from build123d import *

# Parameters (mm, degrees)
EXTRUDE_1_DEPTH     = 26
EXTRUDE_2_DEPTH     = 19
FILLET_1_R          = 10
EXTRUDE_3_DEPTH     = 2
SKETCH_5_W          = 161
SKETCH_5_H          = 6
CUT_EXTRUDE_1_DEPTH = 52
SKETCH_7_W          = 20
SKETCH_7_H          = 20
CUT_EXTRUDE_2_DEPTH = 72
SKETCH_8_W          = 20
SKETCH_8_H          = 20
CUT_EXTRUDE_3_DEPTH = 72
CUT_EXTRUDE_4_DEPTH = 362
SKETCH_9_W          = 9
SKETCH_9_H          = 9
EXTRUDE_4_DEPTH     = 15
EXTRUDE_5_DEPTH     = 20


with BuildPart() as part:
    # Sketch 1 → Extrude 1 (new body)
    with BuildSketch(Plane.XY):
        Polygon((-168, 0), (168, 0), (183, 0), (183, -340), (168, -340), (168, -20), (-168, -20), (-168, -340), (-183, -340), (-183, 0), align=None)
    extrude(amount=EXTRUDE_1_DEPTH)

    # Sketch 1_4 → Extrude 2 (add)
    with BuildSketch(Plane.XY):
        Polygon((172, 0), (168, 0), (168, -20), (168, -340), (172, -340), align=None)
        Polygon((-168, -20), (-168, 0), (-172, 0), (-172, -340), (-168, -340), align=None)
    extrude(amount=-EXTRUDE_2_DEPTH)

    # Fillet 1
    fillet_1_edges = [part.edges().sort_by_distance(p)[0] for p in [
        (170, 0, -19),
        (170, -340, -19),
        (-170, -340, -19),
        (-170, 0, -19),
    ]]
    fillet(fillet_1_edges, radius=FILLET_1_R)

    # Sketch 3 → Extrude 3 (add)
    with BuildSketch(Plane.ZY.offset(-168)):
        with BuildLine():
            Line((-12, -339.539392014), (-12, -0.460607986))
            ThreePointArc((-12, -0.460607986), (-13.02408013, -0.845395743), (-14, -1.339745962))
            Line((-14, -1.339745962), (-14, -338.660254038))
            ThreePointArc((-14, -338.660254038), (-13.02408013, -339.154604257), (-12, -339.539392014))
        make_face()
    extrude_3 = extrude(amount=EXTRUDE_3_DEPTH)

    # Mirror 1: Extrude 3 across plane
    add(extrude_3.mirror(Plane(origin=(0, 0, 0), x_dir=(0, 0, 1), z_dir=(1, 0, 0))))

    # Sketch 5 → Cut-Extrude 1 (cut)
    with BuildSketch(Plane(origin=(0, 0, 0), x_dir=(1, 0, 0), z_dir=(0, 1, 0))):
        with Locations((-87.5, -3)):
            Rectangle(SKETCH_5_W, SKETCH_5_H)
        with Locations((87.5, -3)):
            Rectangle(SKETCH_5_W, SKETCH_5_H)
    extrude(amount=-CUT_EXTRUDE_1_DEPTH, mode=Mode.SUBTRACT)

    # Sketch 7 → Cut-Extrude 2 (cut)
    with BuildSketch(Plane.ZY.offset(-168)):
        with BuildLine():
            Line((26, -340), (26, -20))
            Line((26, -20), (6, -20))
            Line((6, -20), (6, 0))
            Line((6, 0), (-9, 0))
            ThreePointArc((-9, 0), (-10.517576993, -0.115822742), (-12, -0.460607986))
            Line((-12, -0.460607986), (-12, -339.539392014))
            ThreePointArc((-12, -339.539392014), (-10.517576993, -339.884177258), (-9, -340))
            Line((-9, -340), (26, -340))
        make_face()
        with BuildLine():
            Line((-14, -338.660254038), (-14, -1.339745962))
            ThreePointArc((-14, -1.339745962), (-17.660254038, -5), (-19, -10))
            Line((-19, -10), (-19, -330))
            ThreePointArc((-19, -330), (-17.660254038, -335), (-14, -338.660254038))
        make_face()
        with BuildLine():
            ThreePointArc((-12, -0.460607986), (-13.02408013, -0.845395743), (-14, -1.339745962))
            Line((-14, -1.339745962), (-14, -338.660254038))
            ThreePointArc((-14, -338.660254038), (-13.02408013, -339.154604257), (-12, -339.539392014))
            Line((-12, -339.539392014), (-12, -0.460607986))
        make_face()
        with Locations((16, -10)):
            Rectangle(SKETCH_7_W, SKETCH_7_H)
    extrude(amount=-CUT_EXTRUDE_2_DEPTH, mode=Mode.SUBTRACT)


with BuildPart() as cut_extrude_2_piece_1:
    # of the separate pieces the step leaves, piece 1, a body of its own (cut_extrude_2_pieces)
    add(part.part.solids().sort_by_distance((168, 0, 26))[0])

    # Sketch 8 → Cut-Extrude 3 (cut)
    with BuildSketch(Plane(origin=(-168, 0, 0), x_dir=(0, 0, -1), z_dir=(1, 0, 0))):
        with BuildLine():
            Line((9, 0), (-6, 0))
            Line((-6, 0), (-6, -20))
            Line((-6, -20), (-26, -20))
            Line((-26, -20), (-26, -340))
            Line((-26, -340), (9, -340))
            ThreePointArc((9, -340), (10.517576993, -339.884177258), (12, -339.539392014))
            Line((12, -339.539392014), (12, -0.460607986))
            ThreePointArc((12, -0.460607986), (10.517576993, -0.115822742), (9, 0))
        make_face()
        with Locations((-16, -10)):
            Rectangle(SKETCH_8_W, SKETCH_8_H)
    extrude(amount=-CUT_EXTRUDE_3_DEPTH, mode=Mode.SUBTRACT)


with BuildPart() as cut_extrude_2_piece_2:
    # of the separate pieces the step leaves, piece 2, a body of its own (cut_extrude_2_pieces)
    add(part.part.solids().sort_by_distance((168, -339.539392014, -12))[0])


with BuildPart() as cut_extrude_3_piece_1:
    # of the separate pieces the step leaves, piece 1, a body of its own (cut_extrude_3_pieces)
    add(cut_extrude_2_piece_1.part.solids().sort_by_distance((-168, 0, 26))[0])

    # Sketch 9 → Extrude 4 (add)
    with BuildSketch(Plane(origin=(168, 0, 0), x_dir=(0, 0, -1), z_dir=(1, 0, 0))):
        with Locations((-21.5, -15.5)):
            Rectangle(SKETCH_9_W, SKETCH_9_H)
    extrude_4 = extrude(amount=EXTRUDE_4_DEPTH)

    # Mirror 2: Extrude 4 across plane
    add(extrude_4.mirror(Plane(origin=(0, 0, 0), x_dir=(0, 0, 1), z_dir=(1, 0, 0))))

    # Sketch 10 → Extrude 5 (add)
    with BuildSketch(Plane.XY.offset(26)):
        Polygon((168, -20), (162, -20), (168, -26), align=None)
    extrude_5 = extrude(amount=-EXTRUDE_5_DEPTH)

    # Mirror 3: Extrude 5 across plane
    add(extrude_5.mirror(Plane(origin=(0, 0, 0), x_dir=(0, 0, 1), z_dir=(1, 0, 0))))


with BuildPart() as cut_extrude_3_piece_2:
    # of the separate pieces the step leaves, piece 2, a body of its own (cut_extrude_3_pieces)
    add(cut_extrude_2_piece_1.part.solids().sort_by_distance((-172, -0.460607986, -12))[0])


with BuildPart() as cut_extrude_4_tool:
    # Sketch 7_3 → Cut-Extrude 4 (new body)
    with BuildSketch(Plane.ZY.offset(-168)):
        with BuildLine():
            Line((-14, -338.660254038), (-14, -1.339745962))
            ThreePointArc((-14, -1.339745962), (-17.660254038, -5), (-19, -10))
            Line((-19, -10), (-19, -330))
            ThreePointArc((-19, -330), (-17.660254038, -335), (-14, -338.660254038))
        make_face()
        with BuildLine():
            ThreePointArc((-12, -0.460607986), (-13.02408013, -0.845395743), (-14, -1.339745962))
            Line((-14, -1.339745962), (-14, -338.660254038))
            ThreePointArc((-14, -338.660254038), (-13.02408013, -339.154604257), (-12, -339.539392014))
            Line((-12, -339.539392014), (-12, -0.460607986))
        make_face()
    extrude(amount=CUT_EXTRUDE_4_DEPTH)


with BuildPart() as cut_extrude_2_piece_2_1:
    add(cut_extrude_2_piece_2.part)

    # Cut-Extrude 4: cut by cut_extrude_4_tool
    add(cut_extrude_4_tool.part, mode=Mode.SUBTRACT)


with BuildPart() as cut_extrude_3_piece_2_1:
    add(cut_extrude_3_piece_2.part)

    # Cut-Extrude 4: cut by cut_extrude_4_tool
    add(cut_extrude_4_tool.part, mode=Mode.SUBTRACT)


solid = cut_extrude_3_piece_1.part
Verification items for the finished model (mm, model axes). A direction names the side the tool comes from. Coordinates: 2 decimals unless noted, no trailing zeros. Write each loop counter-clockwise with the first axis right and the second up, starting at its lowest first coordinate (ties: lowest second). Pieces come first, ordered by that corner, then holes. Notation, with made-up numbers: M -20.5,43.25 L -7.5,43.25 A25 ccw -7.5,55.25 Z; hole C -2.75,36.25 d5. An arc over 180 degrees is marked long. One line per question, with ' | ' between items.
1) Sectioned sample at A-A on y = -4. Record the cut outline in (x, z), then the cut area to 3 significant figures.
Solutions:
outline: M -168,6 L -7,6 L -7,0 L 7,0 L 7,6 L 168,6 L 168,26 L -168,26 Z | area: 6,800 mm^2
2) Access from +Z, -Z, +X, -X, +Y, -Y to the whole of each face (thin tool, end or side, straight path). Record for faces 5 (the face through (7, -10, 3)), 6 (the face through (176, -20, 22)), 7 (the face through (-86, -10, 6)), 8 (the face through (2, -20, 16)).
Solutions:
face 5: -Z, +X, +Y, -Y | face 6: +Z, -Z, +X, -Y | face 7: -Z, -X, +Y, -Y | face 8: +Z, -Z, -Y
3) Release check for a two-part mould opening along X. For faces 1 (the face through (-175, -20, 22)), 2 (the face through (-183, -15, 22)), 3 (the face through (183, -15, 22)), 4 (the face through (-165, -23, 16)) record: +X half, -X half, draft (parallel to the pull), parting line (faces both ways), or undercut.
Solutions:
face 1: draft | face 2: -X half | face 3: +X half | face 4: undercut
4) Sectioned sample at C-C on x = -141.5. Record the cut outline in (y, z).
Solutions:
outline: M -20,6 L 0,6 L 0,26 L -20,26 Z
5) Sectioned sample at B-B on z = 20.25. Record the cut outline in (x, y).
Solutions:
outline: M -183,-20 L -168,-20 L -168,-26 L -162,-20 L 162,-20 L 168,-26 L 168,-20 L 183,-20 L 183,-11 L 168,-11 L 168,0 L -168,0 L -168,-11 L -183,-11 Z
6) Depth check by flat-ended pin: pin 1 Ø10 at (x, z) = (175, 23) entering from +Y; pin 2 Ø1.5 at (x, y) = (86, -9.5) entering from -Z; pin 3 Ø2 at (y, z) = (-6.5, 21) entering from -X; pin 4 Ø10 at (y, z) = (-21, 19.5) entering from -X. Enter the tip coordinate at first touch or a pass-through.
Solutions:
pin 1: y = -11 | pin 2: z = 6 | pin 3: x = -168 | pin 4: x = -183
7) Material ranges on L1, parallel to Y at x = 102, z = 14.25; L2, parallel to Z at x = 59, y = -17.25; L3, parallel to X at y = -6, z = 6.25, recorded low to high.
Solutions:
L1: -20 to 0 | L2: 6 to 26 | L3: -168 to 168
